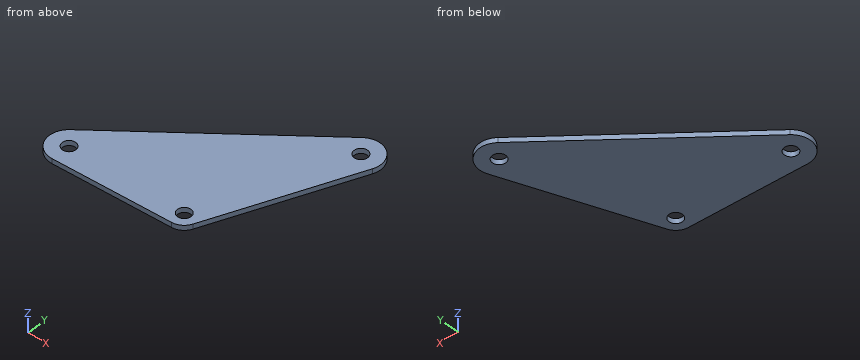
Autodesk Inventor part; units mm, degrees
ref_plane "YZ Plane" through (0, 0, 0) normal (1, 0, 0) x (0, 1, 0)
ref_plane "XZ Plane" through (0, 0, 0) normal (0, 1, 0) x (-1, 0, 0)
ref_plane "XY Plane" through (0, 0, 0) normal (0, 0, 1) x (1, 0, 0)
sketch "main" plane through (0, 0, 0) normal (0, 0, 1) x (1, 0, 0)
  circle A0 centre (29.151, 60.8665) radius 2.1844
  circle A1 centre (29.151, 22.7665) radius 2.1844
  arc A2 (34.0093, 64.9555) -> (22.8065, 60.6019) centre (29.151, 60.8665) ccw
  arc A3 (24.3927, 22.568) -> (27.4035, 18.3362) centre (29.151, 22.7665) ccw
  circle A4 centre (74.9944, 6.3902) radius 2.1844
  arc A5 (72.6644, 0.4831) -> (79.8529, 10.4788) centre (74.9944, 6.3902) ccw
  line L0 (34.0093, 64.9555) -> (79.8529, 10.4788)
  line L1 (22.8065, 60.6019) -> (24.3927, 22.568)
  line L2 (72.6644, 0.4831) -> (27.4035, 18.3362)
  point P0 (-11.6855, 6.8462)
  point P1 (25.2705, 20.0056)
  dimension "d7" = 4.3688
  dimension "d8" = 12.7
  dimension "d9" = 9.525
sketch "Sketch1" plane through (0, 0, 0) normal (0, 0, 1) x (1, 0, 0)
  circle A0 centre (-21.7237, 55.4843) radius 2.1844
  circle A1 centre (16.3762, 55.4424) radius 2.1844
  arc A2 (-25.8074, 60.3471) -> (-21.4661, 49.1395) centre (-21.7237, 55.4843) ccw
  arc A3 (16.5694, 50.6838) -> (20.8046, 53.69) centre (16.3762, 55.4424) ccw
  circle A4 centre (32.803, 101.2677) radius 2.1844
  arc A5 (38.7075, 98.9311) -> (28.7197, 106.1307) centre (32.803, 101.2677) ccw
  line L0 (-25.8074, 60.3471) -> (28.7197, 106.1307)
  line L1 (-21.4661, 49.1395) -> (16.5694, 50.6838)
  line L2 (38.7075, 98.9311) -> (20.8046, 53.69)
extrude "Extrusion2" add sketch "Sketch1" along normal blind 1.5875
properties part number "half_motor_mount" material "Acetal Resin, White"
Can you work these out from the model? Positions are in its coordinate system, mm. Coordinates: 2 decimals unless noted, no trailing zeros. Loops run counter-clockwise (first coordinate to the right, second up) from the corner with the lowest first, then second, coordinate; pieces in that order, holes last. Notation, with made-up numbers: M 74,12.25 L 107,12.25 A12 ccw 107,23.25 Z; hole C -34.5,-19 d5. An arc over 180 degrees is marked long. Return JSON: item names as keys, results as strings. Group by question number.
Item 1: I'm going to push a flat-ended pin straight in: pin 1 Ø6 at (x, y) = (6.5, 91.5) entering from +Z. Where does the tip first touch, or does it pass through?
Item 2: Imagine slicing it at C-C (y = 94.5). Please give me the cut outline in (x, z), and give its area (3 significant figures).
Item 3: Imagine slicing it at B-B (x = -4.5). Please give me the cut outline in (y, z), and give its area (3 significant figures).
Item 4: Imagine slicing it at A-A (z = 0.3). Please give me the cut outline in (x, y).
Item 5: If I drill on L1, parallel to X at y = 54, z = 0.3; L2, parallel to X at y = 58, z = 1.5; L3, parallel to Y at x = 12, z = 1.1, over which ranges is the centre line in solid material (lowest first)? Write a range as from..to.
Verdict:
{
 "1": {"pin 1": "passes through"},
 "2": {"outline": "M 14.87,0 L 36.95,0 L 36.95,1.59 L 14.87,1.59 Z", "area": "35.1 mm^2"},
 "3": {"outline": "M 49.83,0 L 78.24,0 L 78.24,1.59 L 49.83,1.59 Z", "area": "45.1 mm^2"},
 "4": {"outline": "M -25.81,60.35 A6.35 ccw -21.47,49.14 L 16.57,50.68 A4.76 ccw 20.8,53.69 L 38.71,98.93 A6.35 ccw 28.72,106.13 Z; hole C -21.72,55.48 d4.37; hole C 16.38,55.44 d4.37; hole C 32.8,101.27 d4.37"},
 "5": {"L1": "x = -27.9..-23.33, -20.12..14.74, 18.02..20.93", "L2": "x = -27.55..22.51", "L3": "y = 50.5..92.09"}
}
